from build123d import *

# Parameters (mm, degrees)
SKETCH1_W                       = 39.69
SKETCH1_H                       = 39.69
SKETCH1_R                       = 1.75
SKETCH1_R_2                     = 9
BOSS_EXTRUDE1_DEPTH             = 3.175
SKETCH2_R                       = 1.75
BOSS_EXTRUDE2_DEPTH             = 9.635
SKETCH3_W                       = 29.69
SKETCH3_H                       = 6.35
CUT_EXTRUDE1_DEPTH              = 40.69
CBORE_FOR_M3_SBHCS1_D           = 3.4
CBORE_FOR_M3_SBHCS1_DEPTH       = 14.3
CBORE_FOR_M3_SBHCS1_CBORE_D     = 6.7
CBORE_FOR_M3_SBHCS1_CBORE_DEPTH = 1.65
CBORE_FOR_M3_SBHCS1_TIP         = 1.021463052
CBORE_FOR_M3_SBHCS2_AT_2_COUNT  = 2
CBORE_FOR_M3_SBHCS2_AT_2_PITCH  = 30.32
FILLET1_R                       = 3.175
CUT_EXTRUDE2_REACH              = 14.81
SKETCH8_R                       = 2.5


with BuildPart() as part:
    # Sketch1 → Boss-Extrude1 (new body)
    with BuildSketch(Plane(origin=(0, 0, 0), x_dir=(1, 0, 0), z_dir=(0, 1, 0))):
        with Locations((19.845, 19.845)):
            Rectangle(SKETCH1_W, SKETCH1_H)
        with Locations((4.685, 4.685)):
            Circle(SKETCH1_R, mode=Mode.SUBTRACT)
        with Locations((35.005, 4.685)):
            Circle(SKETCH1_R, mode=Mode.SUBTRACT)
        with Locations((35.005, 35.005)):
            Circle(SKETCH1_R, mode=Mode.SUBTRACT)
        with Locations((4.685, 35.005)):
            Circle(SKETCH1_R, mode=Mode.SUBTRACT)
        with Locations((19.845, 19.845)):
            Circle(SKETCH1_R_2, mode=Mode.SUBTRACT)
    extrude(amount=BOSS_EXTRUDE1_DEPTH)

    # Sketch2 → Boss-Extrude2 (add)
    with BuildSketch(Plane(origin=(0, 3.175, 0), x_dir=(1, 0, 0), z_dir=(0, 1, 0))):
        with BuildLine():
            Line((0, 35.005), (0, 39.69))
            Line((0, 39.69), (4.685, 39.69))
            Line((4.685, 39.69), (35.005, 39.69))
            Line((35.005, 39.69), (39.69, 39.69))
            Line((39.69, 39.69), (39.69, 35.005))
            ThreePointArc((39.69, 35.005), (39.441954912, 33.500787212), (38.724084904, 32.15585408))
            Line((38.724084904, 32.15585408), (25.79871116, 15.283933959))
            ThreePointArc((25.79871116, 15.283933959), (19.845, 12.345), (13.89128884, 15.283933959))
            Line((13.89128884, 15.283933959), (0.965915096, 32.15585408))
            ThreePointArc((0.965915096, 32.15585408), (0.248045088, 33.500787212), (0, 35.005))
        make_face()
        with Locations((35.005, 35.005)):
            Circle(SKETCH2_R, mode=Mode.SUBTRACT)
        with Locations((4.685, 35.005)):
            Circle(SKETCH2_R, mode=Mode.SUBTRACT)
    extrude(amount=BOSS_EXTRUDE2_DEPTH)

    # Sketch3 → Cut-Extrude1 (cut, through all)
    with BuildSketch(Plane.ZY):
        with Locations((-14.845, 6.35)):
            Rectangle(SKETCH3_W, SKETCH3_H)
    extrude(amount=-CUT_EXTRUDE1_DEPTH, mode=Mode.SUBTRACT)

    # CBORE for M3 SBHCS1
    with Locations(Plane(origin=(0, 12.81, 0), x_dir=(1, 0, 0), z_dir=(0, 1, 0))):
        with Locations((4.685, 35.005), (35.005, 35.005)):
            CounterBoreHole(CBORE_FOR_M3_SBHCS1_D / 2, CBORE_FOR_M3_SBHCS1_CBORE_D / 2, CBORE_FOR_M3_SBHCS1_CBORE_DEPTH, depth=CBORE_FOR_M3_SBHCS1_DEPTH)
            with Locations((0, 0, -(CBORE_FOR_M3_SBHCS1_DEPTH + CBORE_FOR_M3_SBHCS1_TIP / 2))):  # 118° drill point
                Cone(0, CBORE_FOR_M3_SBHCS1_D / 2, CBORE_FOR_M3_SBHCS1_TIP, mode=Mode.SUBTRACT)

    # Sketch7 → CBORE for M3 SBHCS2 (revolve, cut)
    with BuildSketch(Plane(origin=(4.685, 3.175, -4.685), x_dir=(0, 0, 1), z_dir=(1, 0, 0))):
        Polygon((0, 0), (0, 15.321463052), (1.7, 14.3), (1.7, 1.65), (3.35, 1.65), (3.35, 0.025), (3.375, 0), align=None)
    cbore_for_m3_sbhcs2 = revolve(axis=Axis((4.685, 9.525, -4.685), (0, -1, 0)), mode=Mode.SUBTRACT)

    # CBORE for M3 SBHCS2 at 2: CBORE for M3 SBHCS2 ×2
    with Locations(*[(i * CBORE_FOR_M3_SBHCS2_AT_2_PITCH, 0, 0) for i in range(1, CBORE_FOR_M3_SBHCS2_AT_2_COUNT)]):
        add(cbore_for_m3_sbhcs2, mode=Mode.SUBTRACT)

    # Fillet1
    fillet1_edges = [part.edges().sort_by_distance(p)[0] for p in [
        (0, 6.405, -39.69),
        (39.69, 6.405, -39.69),
        (39.69, 1.5875, 0),
        (0, 1.5875, 0),
    ]]
    fillet(fillet1_edges, radius=FILLET1_R)

    # Sketch8 → Cut-Extrude2 (cut, up to next)
    with BuildSketch(Plane(origin=(0, 12.81, 0), x_dir=(1, 0, 0), z_dir=(0, 1, 0)), mode=Mode.PRIVATE) as cut_extrude2_sk1:
        with Locations((19.845, 19.845)):
            Circle(SKETCH8_R)
    cut_extrude2_tool1 = extrude(cut_extrude2_sk1.sketch, amount=-CUT_EXTRUDE2_REACH, mode=Mode.PRIVATE) & part.part
    add(cut_extrude2_tool1.solids().sort_by_distance((19.845, 12.81, -19.845))[0], mode=Mode.SUBTRACT)


solid = part.part
Work out the finished part from the listing and answer in its coordinate system (mm). A direction names the side the tool comes from. Give positions to 0.01 mm unless a question says otherwise; leave off trailing zeros. Write each loop counter-clockwise with the first axis right and the second up, starting at its lowest first coordinate (ties: lowest second). Pieces come first, ordered by that corner, then holes. Notation, with made-up numbers: M 60.25,-34.75 L 84.25,-34.75 A27 cw 84.25,3.25 Z; hole C 7,14.5 d4. An arc over 180 degrees is marked long. Answer as CSV lines item,"result".
Q1. Given P1, Ø6, axis at x = 19.845, z = -19.845, coming from the +Y side; P2, Ø8.5, axis at x = 19, z = -24, coming from the -Y side (3 decimals); P3, Ø7.5, axis at x = 3.5, z = -3.5, coming from the +Y side (3 decimals); P4, Ø5.5, axis at x = 4.685, z = -35.005, coming from the +Y side, each flat-ended and moving along its own axis, determine where each tip first touches the part or whether it passes through.
A:
P1,"stops at y = 12.81"
P2,"stops at y = 9.525"
P3,"stops at y = 3.175"
P4,"stops at y = 11.16"
Q2. A cutting plane is placed at D-D on y = 1. Write down the section's boundary in (x, z) (3 decimals), plus the area to 3 significant figures.
A:
outline,"M 0,-36.515 A3.175 ccw 3.175,-39.69 L 36.515,-39.69 A3.175 ccw 39.69,-36.515 L 39.69,-3.175 A3.175 ccw 36.515,0 L 3.175,0 A3.175 ccw 0,-3.175 Z; hole C 4.685,-35.005 d3.5; hole C 4.685,-4.685 d3.5; hole C 19.845,-19.845 d18; hole C 35.005,-35.005 d3.5; hole C 35.005,-4.685 d3.5"
area,"1,270 mm²"
Q3. A cutting plane is placed at B-B on z = -34.5. Write down the section's boundary in (x, y) (3 decimals).
A:
outline,"M 0,0 L 3.009,0 L 3.009,11.16 L 1.373,11.16 L 1.373,12.81 L 0.027,12.81 L 0.027,3.175 L 0,3.175 Z; M 6.361,0 L 33.329,0 L 33.329,11.16 L 31.693,11.16 L 31.693,12.81 L 7.997,12.81 L 7.997,11.16 L 6.361,11.16 Z; M 36.681,0 L 39.69,0 L 39.69,3.175 L 39.663,3.175 L 39.663,12.81 L 38.317,12.81 L 38.317,11.16 L 36.681,11.16 Z"
Q4. A tool of negligible diameter and unlimited length cuts with its end or side. For faces 1 (the cylindrical face through (39.45, 7.93, -33.52)), 2 (the cylindrical face through (1.364, 2.349, -5.121)), 3 (the cylindrical face through (13, 2, -14)), from which of +Z, -Z, +X, -X, +Y, -Y can it reach the whole face along a straight path? Write none if from no direction.
A:
face 1,"+Z, +X, +Y"
face 2,"+Y"
face 3,"-Y"
Q5. A cutting plane is placed at A-A on y = 9. Write down the section's boundary in (x, z) (3 decimals).
A:
outline,"M 0,-36.515 A3.175 ccw 3.175,-39.69 L 36.515,-39.69 A3.175 ccw 39.69,-36.515 L 39.69,-35.005 A4.685 ccw 38.724,-32.156 L 36.835,-29.69 L 2.855,-29.69 L 0.966,-32.156 A4.685 ccw 0,-35.005 Z; hole C 4.685,-35.005 d3.5; hole C 35.005,-35.005 d3.5"
Q6. A cutting plane is placed at C-C on x = 23.5. Write down the section's boundary in (y, z) (3 decimals), plus the area to 3 significant figures.
A:
outline,"M 0,-39.69 L 12.81,-39.69 L 12.81,-13.296 L 9.525,-13.296 L 9.525,-29.69 L 3.175,-29.69 L 3.175,-28.069 L 0,-28.069 Z; M 0,-11.621 L 3.175,-11.621 L 3.175,0 L 0,0 Z"
area,"224 mm²"
Q7. The mould has two halves that part along Z. Classify faces 4 (the flat face through (33.788, 10.066, -25.713)), 5 (the cylindrical face through (38.74, 6.32, -38.78)), 6 (the cylindrical face through (3.296, 0.752, -3.62)): +Z half, -Z half, draft (parallel to the pull), parting line (faces both ways), or undercut.
A:
face 4,"+Z half"
face 5,"-Z half"
face 6,"undercut"
Q8. Find the intervals of material crossed by probe 1 along Y at (x, z) = (9, -29.5) (3 decimals); probe 2 along Y at (x, z) = (2.5, -23) (3 decimals); probe 3 along Y at (x, z) = (37, -33.5), in increasing order. Write a range as [from, to].
A:
probe 1,"y = [0, 3.175], [9.525, 12.81]"
probe 2,"y = [0, 3.175]"
probe 3,"y = [0, 11.16]"
